```python
from build123d import *

# Parameters (mm, degrees)
F0_W      = 19
F0_H      = 19.25
F1_DEPTH  = 10
F2_R      = 4
F3_DEPTH  = 8
F4_SIZE2  = 3
F4_SIZE   = 3.5
F5_R      = 3.25
F6_DEPTH  = 2
F8_DEPTH  = 2
F9_SIZE   = 0.5
F10_R     = 1.35
F11_DEPTH = 8


with BuildPart() as f1:
    # F0 (on Top) → F1 (new body)
    with BuildSketch(Plane.XY):
        with Locations((9.5, 9.625)):
            Rectangle(F0_W, F0_H)
    extrude(amount=F1_DEPTH)

    # F2 (on face) → F3 (join)
    with BuildSketch(Plane.XY.offset(10)):
        with Locations((7, 13.25)):
            Circle(F2_R)
    extrude(amount=F3_DEPTH)

    # F4
    f4_edges = [f1.edges().sort_by_distance(p)[0] for p in [
        (3, 13.25, 18),
    ]]
    f4_side = f1.faces().sort_by_distance((7, 13.25, 18))[0]
    chamfer(f4_edges, length=F4_SIZE, length2=F4_SIZE2, reference=f4_side)

    # F5 (on face) → F6 (join)
    with BuildSketch(Plane(origin=(0, 0, 0), x_dir=(0, -1, 0), z_dir=(-1, 0, 0))):
        with Locations((-6.25, 5)):
            Circle(F5_R)
    extrude(amount=F6_DEPTH)

    # F7 (on face) → F8 (join)
    with BuildSketch(Plane.YZ.offset(19)):
        with BuildLine():
            Line((13, 8.5), (6.25, 8.5))
            ThreePointArc((6.25, 8.5), (2.75, 5), (6.25, 1.5))
            Line((6.25, 1.5), (13, 1.5))
            ThreePointArc((13, 1.5), (16.5, 5), (13, 8.5))
        make_face()
    extrude(amount=F8_DEPTH)

    # F9
    f9_edges = [f1.edges().sort_by_distance(p)[0] for p in [
        (19, 19.25, 5),
        (0, 19.25, 5),
        (0, 0, 5),
        (19, 0, 5),
        (0, 9.625, 10),
        (9.5, 19.25, 10),
        (9.5, 0, 10),
        (19, 9.625, 10),
        (3, 13.25, 10),
        (0, 9.5, 5),
        (19, 9.625, 8.5),
    ]]
    chamfer(f9_edges, length=F9_SIZE)

    # F10 (on face) → F11 (cut)
    with BuildSketch(Plane(origin=(0, 0, 0), x_dir=(1, 0, 0), z_dir=(0, 0, -1))):
        with Locations((9.5, -9.625)):
            Circle(F10_R)
    extrude(amount=-F11_DEPTH, mode=Mode.SUBTRACT)


solid = f1.part
```
Build history of the part. All positions in model axes, mm. A direction names the side the tool comes from. Give positions to 0.01 mm unless a question says otherwise; leave off trailing zeros. Loops run counter-clockwise (first coordinate to the right, second up) from the corner with the lowest first, then second, coordinate; pieces in that order, holes last.
1) Band-saw the part on B-B on x = 7. List the corners of the cut face in (y, z), then the cut area to 3 significant figures.
Values follow:
outline: (0, 0) - (19.25, 0) - (19.25, 9.5) - (18.75, 10) - (17.75, 10) - (17.25, 10.5) - (17.25, 15) - (13.75, 18) - (12.75, 18) - (9.25, 15) - (9.25, 10.5) - (8.75, 10) - (0.5, 10) - (0, 9.5) - close
area: 246 mm2
2) Band-saw the part on C-C on x = 12. List the corners of the cut face in (y, z), then the cut area to 3 significant figures.
Values follow:
outline: (0, 0) - (19.25, 0) - (19.25, 9.5) - (18.75, 10) - (0.5, 10) - (0, 9.5) - close
area: 192 mm2
3) Drop flat-ended pins along their axis: P1, Ø2, axis at y = 12.5, z = 6, coming from the -X side; P2, Ø10, axis at x = 3.5, y = 11.5, coming from the -Z side; P3, Ø2, axis at x = 9.5, y = 9.5, coming from the -Z side; P4, Ø3.5, axis at x = 9.5, y = 9.625, coming from the +Z side. Give the stop position or say it passes through.
Values follow:
P1: stops at x = 0
P2: stops at z = 0
P3: stops at z = 8
P4: stops at z = 16.15
4) 3-axis set-ups, long thin cutter, end or side, ignore diameter. For faces 4 (the face through (20.24, 2.75, 5.08)), 5 (the face through (20, 10, 1.5)), 6 (the face through (9, 19.25, 5)), 7 (the face through (-1.24, 3.15, 5.98)), 8 (the face through (10.23, 8.49, 3.94)): which of +Z, -Z, +X, -X, +Y, -Y reach the whole face in a straight line?
Values follow:
face 4: +X, -Y
face 5: -Z, +X, +Y, -Y
face 6: +Z, -Z, +X, -X, +Y
face 7: -X
face 8: -Z
5) Probe line 1 along Y through (x, z) = (9.5, 1.75) (3 decimals); line 2 along X through (y, z) = (13, 13); line 3 along X through (y, z) = (1.75, 5.5). List the from-to ranges inside material, lowest first.
Values follow:
line 1: y = 0 to 8.275, 10.975 to 19.25
line 2: x = 3.01 to 10.99
line 3: x = 0 to 19
6) Two-plate mould, pull along Y, no slides. Class faces 1 (the face through (9, 10, 8)), 2 (the face through (6.479, 17.216, 12.718)), 3 (the face through (20.2, 16.5, 4.9)): released by +Y, released by -Y, zero draft, split by the parting line, or undercut.
Values follow:
face 1: undercut
face 2: split by the parting line
face 3: released by +Y
7) Band-saw the part on A-A on z = 5. List the corners of the cut face in (x, y) (3 decimals), then the cut area to 3 significant figures.
Values follow:
outline: (-2, 3) - (-0.5, 3) - (0, 2.5) - (0, 0.5) - (0.5, 0) - (18.5, 0) - (19, 0.5) - (19, 2.25) - (19.5, 2.75) - (21, 2.75) - (21, 16.5) - (19.5, 16.5) - (19, 17) - (19, 18.75) - (18.5, 19.25) - (0.5, 19.25) - (0, 18.75) - (0, 10) - (-0.5, 9.5) - (-2, 9.5) - close; hole circle Ø2.7 at (9.5, 9.625)
area: 401 mm2
